Work out the finished part from the listing and answer in its coordinate system (mm). A direction names the side the tool comes from. Coordinates: 2 decimals unless noted, no trailing zeros. Loops run counter-clockwise (first coordinate to the right, second up) from the corner with the lowest first, then second, coordinate; pieces in that order, holes last. Notation, with made-up numbers: (74.5, 88.5) - (129.5, 88.5) arc R21 cw to (129.5, 94.5) - close; hole circle Ø7 at (5.25, -25.75). An arc over 180 degrees is marked (long way). Write each question's results on one line, items separated by ' | '. Start each with the question number.
1. A cutting plane is placed at D-D on x = 26. Determine the outline of the cut face in (y, z), then the cut area to 3 significant figures.
2. Which of the six approach directions +Z, -Z, +X, -X, +Y, -Y give full straight-line access (tool end or side, diameter ignored) to faces 1 (the cylindrical face through (-58.78, 57.89, 1.48)), 2 (the cylindrical face through (-74.044, 48.281, 8.409)), 3 (the flat face through (2, -99, 15))?
3. Find the intervals of material crossed by line 1 along Y through (x, z) = (0, 12.5); line 2 along X through (y, z) = (0.5, 10.25); line 3 along Y through (x, z) = (-47.5, 1.5), in increasing order. Write a range as [from, to].
4. Each of these flat-tipped pins is pushed along its axis until it touches: P1, Ø3.5, axis at x = -60, z = 1, coming from the +Y side; P2, Ø4, axis at x = -10.5, z = 11, coming from the +Y side; P3, Ø3.5, axis at y = 60, z = 2, coming from the +X side; P4, Ø4, axis at x = -26.5, z = 6.5, coming from the +Y side. Where does it stop, or does it pass through?
5. A cutting plane is placed at A-A on x = 0. State how many separate pieces and enclosed holes the cut face has, then the cut area to 3 significant figures.
6. Determine the mould class of faces 4 (the flat face through (-78, 40, 15)), 5 (the flat face through (-46, -80, 2)) for opening direction X: released by +X, released by -X, zero draft, split by the parting line, or undercut.
from build123d import *

# Parameters (mm, degrees)
F0_R     = 102.5
F0_R_2   = 9.5
F0_W     = 52.984908
F0_H     = 6.946532
F0_W_2   = 6.946532
F0_H_2   = 52.984908
F1_DEPTH = 3
F0_R_3   = 6.5
F2_DEPTH = 15
F3_DEPTH = 2


with BuildPart() as f1:
    # F0 (on Top) → F1 (new body)
    with BuildSketch(Plane.XY):
        Circle(F0_R)
        with Locations((-46.328817, -80.243864)):
            Circle(F0_R_2, mode=Mode.SUBTRACT)
        with Locations((-80.243864, -46.328817)):
            Circle(F0_R_2, mode=Mode.SUBTRACT)
        with Locations((0, -92.657633)):
            Circle(F0_R_2, mode=Mode.SUBTRACT)
        with Locations((46.328817, -80.243864)):
            Circle(F0_R_2, mode=Mode.SUBTRACT)
        with Locations((80.243864, -46.328817)):
            Circle(F0_R_2, mode=Mode.SUBTRACT)
        with Locations((-92.657633, 0)):
            Circle(F0_R_2, mode=Mode.SUBTRACT)
        with Locations((-80.243864, 46.328817)):
            Circle(F0_R_2, mode=Mode.SUBTRACT)
        with Locations((-46.328817, 80.243864)):
            Circle(F0_R_2, mode=Mode.SUBTRACT)
        with BuildLine():
            ThreePointArc((80.074814, 19.856338), (81.891459, 10.001946), (82.5, 0))
            ThreePointArc((82.5, 0), (81.891459, -10.001946), (80.074814, -19.856338))
            ThreePointArc((80.074814, -19.856338), (58.336309, -58.336309), (19.856338, -80.074814))
            ThreePointArc((19.856338, -80.074814), (0, -82.5), (-19.856338, -80.074814))
            ThreePointArc((-19.856338, -80.074814), (-58.336309, -58.336309), (-80.074814, -19.856338))
            ThreePointArc((-80.074814, -19.856338), (-82.5, 0), (-80.074814, 19.856338))
            ThreePointArc((-80.074814, 19.856338), (-58.336309, 58.336309), (-19.856338, 80.074814))
            ThreePointArc((-19.856338, 80.074814), (0, 82.5), (19.856338, 80.074814))
            ThreePointArc((19.856338, 80.074814), (58.336309, 58.336309), (80.074814, 19.856338))
        make_face(mode=Mode.SUBTRACT)
        with Locations((92.657633, 0)):
            Circle(F0_R_2, mode=Mode.SUBTRACT)
        with Locations((80.243864, 46.328817)):
            Circle(F0_R_2, mode=Mode.SUBTRACT)
        with Locations((0, 92.657633)):
            Circle(F0_R_2, mode=Mode.SUBTRACT)
        with Locations((46.328817, 80.243864)):
            Circle(F0_R_2, mode=Mode.SUBTRACT)
        with Locations((-48.197031, 0)):
            Rectangle(F0_W, F0_H)
        with BuildLine():
            ThreePointArc((-15.717052, 9.093692), (-48.690174, 9.725664), (-80.074814, 19.856338))
            ThreePointArc((-80.074814, 19.856338), (-82.5, 0), (-80.074814, -19.856338))
            ThreePointArc((-80.074814, -19.856338), (-48.690174, -9.725664), (-15.717052, -9.093692))
            ThreePointArc((-15.717052, -9.093692), (-18.15822, 0), (-15.717052, 9.093692))
        make_face()
        with Locations((-48.197031, 0)):
            Rectangle(F0_W, F0_H, mode=Mode.SUBTRACT)
        with BuildLine():
            ThreePointArc((-11.569649, 9.703259), (-13.640522, 9.379231), (-15.717052, 9.093692))
            ThreePointArc((-15.717052, 9.093692), (-18.15822, 0), (-15.717052, -9.093692))
            ThreePointArc((-15.717052, -9.093692), (-13.640522, -9.379231), (-11.569649, -9.703259))
            ThreePointArc((-11.569649, -9.703259), (-15.1, 0), (-11.569649, 9.703259))
        make_face()
        with BuildLine():
            ThreePointArc((-9.703259, 11.569649), (-9.379231, 13.640522), (-9.093692, 15.717052))
            ThreePointArc((-9.093692, 15.717052), (-12.8398, 12.8398), (-15.717052, 9.093692))
            ThreePointArc((-15.717052, 9.093692), (-13.640522, 9.379231), (-11.569649, 9.703259))
            ThreePointArc((-11.569649, 9.703259), (-10.677312, 10.677312), (-9.703259, 11.569649))
        make_face()
        with BuildLine():
            ThreePointArc((9.703259, 11.569649), (9.379231, 13.640522), (9.093692, 15.717052))
            ThreePointArc((9.093692, 15.717052), (0, 18.15822), (-9.093692, 15.717052))
            ThreePointArc((-9.093692, 15.717052), (-9.379231, 13.640522), (-9.703259, 11.569649))
            ThreePointArc((-9.703259, 11.569649), (0, 15.1), (9.703259, 11.569649))
        make_face()
        with BuildLine():
            ThreePointArc((11.569649, 9.703259), (13.640522, 9.379231), (15.717052, 9.093692))
            ThreePointArc((15.717052, 9.093692), (12.8398, 12.8398), (9.093692, 15.717052))
            ThreePointArc((9.093692, 15.717052), (9.379231, 13.640522), (9.703259, 11.569649))
            ThreePointArc((9.703259, 11.569649), (10.677312, 10.677312), (11.569649, 9.703259))
        make_face()
        with BuildLine():
            ThreePointArc((18.15822, 0), (17.537312, 4.707827), (15.717052, 9.093692))
            ThreePointArc((15.717052, 9.093692), (13.640522, 9.379231), (11.569649, 9.703259))
            ThreePointArc((11.569649, 9.703259), (14.189991, 5.162766), (15.1, 0))
            ThreePointArc((15.1, 0), (14.189991, -5.162766), (11.569649, -9.703259))
            ThreePointArc((11.569649, -9.703259), (13.640522, -9.379231), (15.717052, -9.093692))
            ThreePointArc((15.717052, -9.093692), (17.537312, -4.707827), (18.15822, 0))
        make_face()
        with BuildLine():
            ThreePointArc((80.074814, -19.856338), (81.891459, -10.001946), (82.5, 0))
            ThreePointArc((82.5, 0), (81.891459, 10.001946), (80.074814, 19.856338))
            ThreePointArc((80.074814, 19.856338), (48.690174, 9.725664), (15.717052, 9.093692))
            ThreePointArc((15.717052, 9.093692), (17.537312, 4.707827), (18.15822, 0))
            ThreePointArc((18.15822, 0), (17.537312, -4.707827), (15.717052, -9.093692))
            ThreePointArc((15.717052, -9.093692), (48.690174, -9.725664), (80.074814, -19.856338))
        make_face()
        with Locations((48.197031, 0)):
            Rectangle(F0_W, F0_H, mode=Mode.SUBTRACT)
        with BuildLine():
            ThreePointArc((-19.856338, -80.074814), (0, -82.5), (19.856338, -80.074814))
            ThreePointArc((19.856338, -80.074814), (9.725664, -48.690174), (9.093692, -15.717052))
            ThreePointArc((9.093692, -15.717052), (0, -18.15822), (-9.093692, -15.717052))
            ThreePointArc((-9.093692, -15.717052), (-9.725664, -48.690174), (-19.856338, -80.074814))
        make_face()
        with Locations((0, -48.197031)):
            Rectangle(F0_W_2, F0_H_2, mode=Mode.SUBTRACT)
        with BuildLine():
            ThreePointArc((-9.093692, -15.717052), (0, -18.15822), (9.093692, -15.717052))
            ThreePointArc((9.093692, -15.717052), (9.379231, -13.640522), (9.703259, -11.569649))
            ThreePointArc((9.703259, -11.569649), (0, -15.1), (-9.703259, -11.569649))
            ThreePointArc((-9.703259, -11.569649), (-9.379231, -13.640522), (-9.093692, -15.717052))
        make_face()
        with BuildLine():
            ThreePointArc((9.093692, -15.717052), (12.8398, -12.8398), (15.717052, -9.093692))
            ThreePointArc((15.717052, -9.093692), (13.640522, -9.379231), (11.569649, -9.703259))
            ThreePointArc((11.569649, -9.703259), (10.677312, -10.677312), (9.703259, -11.569649))
            ThreePointArc((9.703259, -11.569649), (9.379231, -13.640522), (9.093692, -15.717052))
        make_face()
        with BuildLine():
            ThreePointArc((-15.717052, -9.093692), (-12.8398, -12.8398), (-9.093692, -15.717052))
            ThreePointArc((-9.093692, -15.717052), (-9.379231, -13.640522), (-9.703259, -11.569649))
            ThreePointArc((-9.703259, -11.569649), (-10.677312, -10.677312), (-11.569649, -9.703259))
            ThreePointArc((-11.569649, -9.703259), (-13.640522, -9.379231), (-15.717052, -9.093692))
        make_face()
        with BuildLine():
            ThreePointArc((9.093692, 15.717052), (9.725664, 48.690174), (19.856338, 80.074814))
            ThreePointArc((19.856338, 80.074814), (0, 82.5), (-19.856338, 80.074814))
            ThreePointArc((-19.856338, 80.074814), (-9.725664, 48.690174), (-9.093692, 15.717052))
            ThreePointArc((-9.093692, 15.717052), (0, 18.15822), (9.093692, 15.717052))
        make_face()
        with Locations((0, 48.197031)):
            Rectangle(F0_W_2, F0_H_2, mode=Mode.SUBTRACT)
    extrude(amount=F1_DEPTH)

    # F0 (on Top) → F2 (join)
    with BuildSketch(Plane.XY):
        with Locations((80.243864, 46.328817)):
            Circle(F0_R_2)
        with Locations((80.243864, 46.328817)):
            Circle(F0_R_3, mode=Mode.SUBTRACT)
        with Locations((92.657633, 0)):
            Circle(F0_R_2)
        with Locations((92.657633, 0)):
            Circle(F0_R_3, mode=Mode.SUBTRACT)
        with Locations((80.243864, -46.328817)):
            Circle(F0_R_2)
        with Locations((80.243864, -46.328817)):
            Circle(F0_R_3, mode=Mode.SUBTRACT)
        with Locations((46.328817, -80.243864)):
            Circle(F0_R_2)
        with Locations((46.328817, -80.243864)):
            Circle(F0_R_3, mode=Mode.SUBTRACT)
        with Locations((0, -92.657633)):
            Circle(F0_R_2)
        with Locations((0, -92.657633)):
            Circle(F0_R_3, mode=Mode.SUBTRACT)
        with Locations((-46.328817, -80.243864)):
            Circle(F0_R_2)
        with Locations((-46.328817, -80.243864)):
            Circle(F0_R_3, mode=Mode.SUBTRACT)
        with Locations((-80.243864, -46.328817)):
            Circle(F0_R_2)
        with Locations((-80.243864, -46.328817)):
            Circle(F0_R_3, mode=Mode.SUBTRACT)
        with Locations((-92.657633, 0)):
            Circle(F0_R_2)
        with Locations((-92.657633, 0)):
            Circle(F0_R_3, mode=Mode.SUBTRACT)
        with Locations((-80.243864, 46.328817)):
            Circle(F0_R_2)
        with Locations((-80.243864, 46.328817)):
            Circle(F0_R_3, mode=Mode.SUBTRACT)
        with Locations((46.328817, 80.243864)):
            Circle(F0_R_2)
        with Locations((46.328817, 80.243864)):
            Circle(F0_R_3, mode=Mode.SUBTRACT)
        with Locations((0, 92.657633)):
            Circle(F0_R_2)
        with Locations((0, 92.657633)):
            Circle(F0_R_3, mode=Mode.SUBTRACT)
        with Locations((-46.328817, 80.243864)):
            Circle(F0_R_2)
        with Locations((-46.328817, 80.243864)):
            Circle(F0_R_3, mode=Mode.SUBTRACT)
    extrude(amount=F2_DEPTH)

    # F0 (on Top) → F3 (join)
    with BuildSketch(Plane.XY):
        with Locations((0, 92.657633)):
            Circle(F0_R_3)
        with Locations((46.328817, 80.243864)):
            Circle(F0_R_3)
        with Locations((80.243864, 46.328817)):
            Circle(F0_R_3)
        with Locations((92.657633, 0)):
            Circle(F0_R_3)
        with Locations((80.243864, -46.328817)):
            Circle(F0_R_3)
        with Locations((46.328817, -80.243864)):
            Circle(F0_R_3)
        with Locations((0, -92.657633)):
            Circle(F0_R_3)
        with Locations((-46.328817, -80.243864)):
            Circle(F0_R_3)
        with Locations((-80.243864, -46.328817)):
            Circle(F0_R_3)
        with Locations((-92.657633, 0)):
            Circle(F0_R_3)
        with Locations((-80.243864, 46.328817)):
            Circle(F0_R_3)
        with Locations((-46.328817, 80.243864)):
            Circle(F0_R_3)
    extrude(amount=F3_DEPTH)


solid = f1.part
Values:
1) outline: (-99.15, 0) - (-78.3, 0) - (-78.3, 3) - (-99.15, 3) - close; (-8.25, 0) - (-3.47, 0) - (-3.47, 3) - (-8.25, 3) - close; (3.47, 0) - (8.25, 0) - (8.25, 3) - (3.47, 3) - close; (78.3, 0) - (99.15, 0) - (99.15, 3) - (78.3, 3) - close | area: 154 mm^2
2) face 1: +Z, -Z | face 2: +Z | face 3: +Z, +X, -X, +Y, -Y
3) line 1: [-102.16, -99.16], [-86.16, -83.16], [83.16, 86.16], [99.16, 102.16] | line 2: [-102.14, -99.14], [-86.18, -83.17], [83.17, 86.18], [99.14, 102.14] | line 3: [-90.83, -67.45], [-9.53, -3.47], [3.47, 9.53], [67.45, 90.83]
4) P1: y = 84.34 | P2: y = 96.9 | P3: x = 84.34 | P4: through
5) separate pieces: 4 | enclosed holes: 0 | area: 324 mm^2
6) face 4: zero draft | face 5: undercut
